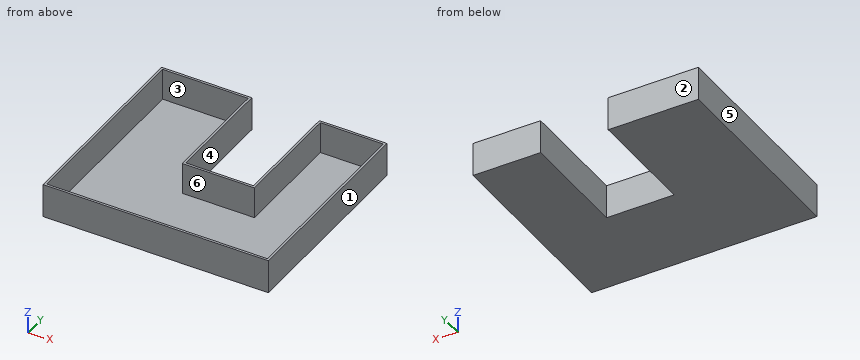
Autodesk Inventor part; units mm, degrees
ref_plane "YZ Plane" through (0, 0, 0) normal (1, 0, 0) x (0, 1, 0)
ref_plane "XZ Plane" through (0, 0, 0) normal (0, 1, 0) x (-1, 0, 0)
ref_plane "XY Plane" through (0, 0, 0) normal (0, 0, 1) x (1, 0, 0)
sketch "Sketch1" plane through (0, 0, 0) normal (0, 0, 1) x (1, 0, 0)
  line L0 (0, 0) -> (-50, 0) construction
  line L1 (0, 0) -> (50, 0) construction
  line L2 (-50, 0) -> (50, 0)
  line L3 (-50, 0) -> (-50, 90)
  line L4 (-79, 0) -> (-79, 40) construction
  line L5 (-79, 40) -> (-79, 90) construction
  line L6 (-50, 90) -> (-10, 90)
  line L7 (-50, 100.5212) -> (20, 100.5212) construction
  line L8 (-10, 90) -> (-10, 40)
  line L9 (-10, 40) -> (20, 40)
  line L10 (20, 40) -> (20, 90)
  line L11 (20, 90) -> (50, 90)
  line L12 (50, 90) -> (50, 0)
  dimension "d2" = 90
  dimension "d3" = 40
  dimension "d4" = 50
  dimension "d5" = 40
  dimension "d6" = 70
extrude "Extrusion1" add sketch "Sketch1" along normal blind 15
shell "Shell1" thickness 1 removed faces 1 at (-3.3333, 13.3333, 15)
properties part number "shim_3DPrint"
Can you work these out from the model? Positions are in its coordinate system, mm. Face numbers are marked on the shaded views. A direction names the side the tool comes from. Give positions to 0.01 mm unless a question says otherwise; leave off trailing zeros. Loops run counter-clockwise (first coordinate to the right, second up) from the corner with the lowest first, then second, coordinate; pieces in that order, holes last. Notation, with made-up numbers: (66.5, 67.25) -> (71.5, 67.25) arc R16 cw to (71.5, 81.25) -> close; hole circle Ø2 at (-22, 17). An arc over 180 degrees is marked (long way). Write item = value, one per line.
1) I need wall thicknesses on L1, parallel to X at y = 54, z = 14; L2, parallel to Y at x = -16.5, z = 12; L3, parallel to X at y = 20, z = 6.75. Which ranges of each line are inside material? Lowest first, please. Write a range as from..to.
Check result:
L1 = -50..-49, -11..-10, 20..21, 49..50
L2 = 0..1, 89..90
L3 = -50..-49, 49..50
2) Will these pins go through, and if not, where does the flat tip stop? pin 1 (8 mm diameter, centred on x = 26, y = 41, fed in from -Z); pin 2 (7.5 mm diameter, centred on x = -0.5, z = 7, fed in from +Y); pin 3 (6 mm diameter, centred on x = -30, y = 49.5, fed in from +Z).
Check result:
pin_1 = 0
pin_2 = 40
pin_3 = 1
3) Suppose I cut it at A-A on y = 49.5. Write out the boundary of the cut face in (x, z), then the cut area to 3 significant figures.
Check result:
outline = (-50, 0) -> (-10, 0) -> (-10, 15) -> (-11, 15) -> (-11, 1) -> (-49, 1) -> (-49, 15) -> (-50, 15) -> close; (20, 0) -> (50, 0) -> (50, 15) -> (49, 15) -> (49, 1) -> (21, 1) -> (21, 15) -> (20, 15) -> close
area = 126 mm2
4) Suppose I cut it at B-B on z = 5. Write out the boundary of the cut face in (x, y).
Check result:
outline = (-50, 0) -> (50, 0) -> (50, 90) -> (20, 90) -> (20, 40) -> (-10, 40) -> (-10, 90) -> (-50, 90) -> close; hole (-49, 1) -> (49, 1) -> (49, 89) -> (21, 89) -> (21, 39) -> (-11, 39) -> (-11, 89) -> (-49, 89) -> close
5) For the marked faces 4, 5 and 6, which set-ups out of +Z, -Z, +X, -X, +Y, -Y let a thin tool reach every point of the face, with its end or its side?
Check result:
face_4 = +Z, -Z, +Y
face_5 = +Z, -Z, -X, +Y, -Y
face_6 = +Z
6) Thinking about a two-plate mould opening in Y: for the marked faces 1, 2 and 3, which applies, released by +Y, released by -Y, zero draft, split by the parting line, or undercut?
Check result:
face_1 = zero draft
face_2 = released by +Y
face_3 = undercut
7) Suppose I cut it at D-D on y = 35. Write out the boundary of the cut face in (x, z).
Check result:
outline = (-50, 0) -> (50, 0) -> (50, 15) -> (49, 15) -> (49, 1) -> (-49, 1) -> (-49, 15) -> (-50, 15) -> close
8) Suppose I cut it at C-C on x = 1. Write out the boundary of the cut face in (y, z).
Check result:
outline = (0, 0) -> (40, 0) -> (40, 15) -> (39, 15) -> (39, 1) -> (1, 1) -> (1, 15) -> (0, 15) -> close
